Model file for the job. Use its own axes, mm. Coordinates: 2 decimals unless noted, no trailing zeros. Write each loop counter-clockwise with the first axis right and the second up, starting at its lowest first coordinate (ties: lowest second). Pieces come first, ordered by that corner, then holes.
Q1. Drill centre lines: probe 1 along X at (y, z) = (545, 8); probe 2 along Y at (x, z) = (-125, 9.25); probe 3 along Y at (x, z) = (-94, 8). Where is each one in solid material? Low to high.
Q2. Band-saw the part on D-D, the plane y = 595. Write the cut outline in (x, z), plus the area to 3 significant figures.
Q3. Band-saw the part on B-B, the plane z = 3. State how many separate pieces and enclosed holes the cut face has, plus the area to 3 significant figures.
Q4. Band-saw the part on C-C, the plane y = 490. Write the cut outline in (x, z), plus the area to 3 significant figures.
Q5. Pin check, flat tips, straight feed: P1, Ø1.2, axis at y = 595, z = 16, coming from the +X side; P2, Ø8, axis at x = -150.5, z = 5.5, coming from the -Y side (3 decimals); P3, Ø2.5, axis at x = -116.5, y = 593, coming from the +Z side. Stop position of each tip, or through.
Q6. Band-saw the part on A-A, the plane x = -125. Write the cut outline in (y, z), plus the area to 3 significant figures.
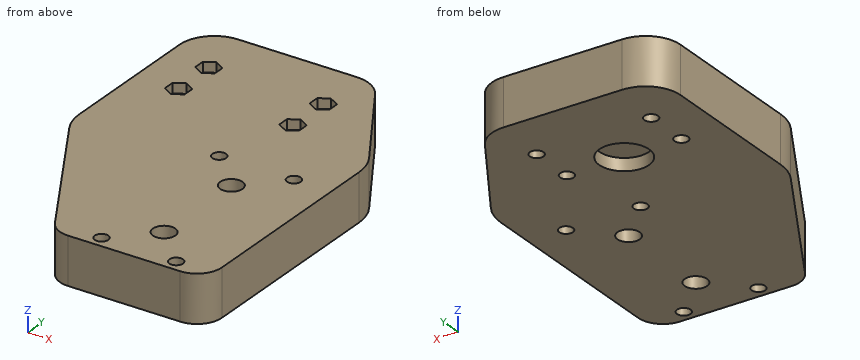
from build123d import *

# Parameters (mm, degrees)
BOSS_EXTRUDE1_DEPTH  = 19
FILLET1_R            = 10
M5_CLEARANCE_HOLE2_D = 5.5
M5_CLEARANCE_HOLE1_D = 5.5
FILLET2_R            = 4
BOSS_EXTRUDE2_DEPTH  = 19
M8_CLEARANCE_HOLE1_D = 9
CUT_EXTRUDE2_DEPTH   = 4
SKETCH16_R           = 10
CUT_EXTRUDE3_DEPTH   = 5


with BuildPart() as part:
    # Sketch1 → Boss-Extrude1 (new body)
    with BuildSketch(Plane.XY):
        with BuildLine():
            Line((-170.200000001, 540.824594888), (-129.309401077, 470))
            Line((-129.309401077, 470), (-93, 470))
            ThreePointArc((-93, 470), (-90.878679656, 470.878679656), (-90, 473))
            Line((-90, 473), (-90, 564.25527297))
            Line((-90, 564.25527297), (-116.225329238, 607))
            Line((-116.225329238, 607), (-170.200000001, 607))
            Line((-170.200000001, 607), (-170.200000001, 540.824594888))
        make_face()
    extrude(amount=BOSS_EXTRUDE1_DEPTH)

    # Fillet1
    fillet1_edges = [part.edges().sort_by_distance(p)[0] for p in [
        (-90, 564.25527297, 9.5),
        (-129.309401077, 470, 9.5),
        (-170.200000001, 540.824594888, 9.5),
    ]]
    fillet(fillet1_edges, radius=FILLET1_R)

    # M5 Clearance Hole2 (through all)
    with Locations(Plane(origin=(0, 0, 0), x_dir=(-1, 0, 0), z_dir=(0, 0, -1))):
        with Locations((117.000000001, 595), (117.000000001, 577), (163.000000001, 577), (163.000000001, 595)):
            Hole(M5_CLEARANCE_HOLE2_D / 2)

    # M5 Clearance Hole1 (through all)
    with Locations(Plane.XY.offset(19)):
        with Locations((-95, 545), (-125, 545), (-125, 475), (-95, 475), (-110, 490), (-110, 530)):
            Hole(M5_CLEARANCE_HOLE1_D / 2)

    # Fillet2
    fillet2_edges = [part.edges().sort_by_distance(p)[0] for p in [
        (-116.225329238, 607, 9.5),
        (-170.200000001, 607, 9.5),
    ]]
    fillet(fillet2_edges, radius=FILLET2_R)

    # Sketch11 → Boss-Extrude2 (add)
    with BuildSketch(Plane.XY.offset(19)):
        with BuildLine():
            ThreePointArc((-143.743157806, 475), (-140.082903769, 471.339745962), (-135.082903769, 470))
            Line((-135.082903769, 470), (-123.535898385, 470))
            ThreePointArc((-123.535898385, 470), (-128.535898385, 471.339745962), (-132.196152423, 475))
            Line((-132.196152423, 475), (-168.860254039, 538.504086813))
            ThreePointArc((-168.860254039, 538.504086813), (-169.859258264, 540.915896362), (-170.200000001, 543.504086813))
            Line((-170.200000001, 543.504086813), (-170.200000001, 603))
            ThreePointArc((-170.200000001, 603), (-169.028427125, 605.828427125), (-166.200000001, 607))
            Line((-166.200000001, 607), (-118.464037729, 607))
            ThreePointArc((-118.464037729, 607), (-116.510482263, 606.490504411), (-115.054590744, 605.091810521))
            Line((-115.054590744, 605.091810521), (-91.476382537, 566.661632408))
            ThreePointArc((-91.476382537, 566.661632408), (-90.37617086, 564.149073659), (-90, 561.432106106))
            Line((-90, 561.432106106), (-90, 473))
            ThreePointArc((-90, 473), (-90.878679656, 470.878679656), (-93, 470))
            Line((-93, 470), (-90, 470))
            ThreePointArc((-90, 470), (-82.928932188, 472.928932188), (-80, 480))
            Line((-80, 480), (-80, 561.432106106))
            ThreePointArc((-80, 561.432106106), (-80.75234172, 566.866041212), (-82.952765074, 571.89115871))
            Line((-82.952765074, 571.89115871), (-106.530973281, 610.321336823))
            ThreePointArc((-106.530973281, 610.321336823), (-111.626593598, 615.216765438), (-118.464037729, 617))
            Line((-118.464037729, 617), (-166.200000001, 617))
            ThreePointArc((-166.200000001, 617), (-176.099494937, 612.899494937), (-180.200000001, 603))
            Line((-180.200000001, 603), (-180.200000001, 543.504086813))
            ThreePointArc((-180.200000001, 543.504086813), (-179.518516526, 538.327705911), (-177.520508076, 533.504086813))
            Line((-177.520508076, 533.504086813), (-143.743157806, 475))
        make_face()
    extrude(amount=-BOSS_EXTRUDE2_DEPTH)

    # M8 Clearance Hole1 (through all)
    with Locations(Plane.XY.offset(19)):
        with Locations((-110, 530), (-110, 490)):
            Hole(M8_CLEARANCE_HOLE1_D / 2)

    # Sketch15 → Cut-Extrude2 (cut)
    with BuildSketch(Plane.XY.offset(19)):
        Polygon((-166.960000001, 579.286307066), (-166.960000001, 574.713692934), (-163.000000001, 572.427385868), (-159.040000001, 574.713692934), (-159.040000001, 579.286307066), (-163.000000001, 581.572614132), align=None)
        Polygon((-120.960000001, 579.286307066), (-120.960000001, 574.713692934), (-117.000000001, 572.427385868), (-113.040000001, 574.713692934), (-113.040000001, 579.286307066), (-117.000000001, 581.572614132), align=None)
        Polygon((-113.040000001, 592.713692934), (-117.000000001, 590.427385868), (-120.960000001, 592.713692934), (-120.960000001, 597.286307066), (-117.000000001, 599.572614132), (-113.040000001, 597.286307066), align=None)
        Polygon((-163.000000001, 590.427385868), (-166.960000001, 592.713692934), (-166.960000001, 597.286307066), (-163.000000001, 599.572614132), (-159.040000001, 597.286307066), (-159.040000001, 592.713692934), align=None)
    extrude(amount=-CUT_EXTRUDE2_DEPTH, mode=Mode.SUBTRACT)

    # Sketch16 → Cut-Extrude3 (cut)
    with BuildSketch(Plane(origin=(0, 0, 0), x_dir=(-1, 0, 0), z_dir=(0, 0, -1))):
        with Locations((140.000000001, 577)):
            Circle(SKETCH16_R)
    extrude(amount=-CUT_EXTRUDE3_DEPTH, mode=Mode.SUBTRACT)


solid = part.part
Answer sheet:
1. probe 1: x = -180.2 to -127.75, -122.25 to -97.75, -92.25 to -80
1. probe 2: y = 470 to 472.25, 477.75 to 542.25, 547.75 to 617
1. probe 3: y = 470 to 472.44, 477.56 to 542.44, 547.56 to 589.9
2. outline: (-180.2, 0) - (-165.75, 0) - (-165.75, 15) - (-166.96, 15) - (-166.96, 19) - (-180.2, 19) - close; (-160.25, 0) - (-119.75, 0) - (-119.75, 15) - (-120.96, 15) - (-120.96, 19) - (-159.04, 19) - (-159.04, 15) - (-160.25, 15) - close; (-114.25, 0) - (-97.13, 0) - (-97.13, 19) - (-113.04, 19) - (-113.04, 15) - (-114.25, 15) - close
2. area: 1,350 mm2
3. separate pieces: 1
3. enclosed holes: 11
3. area: 11,900 mm2
4. outline: (-152.4, 0) - (-114.5, 0) - (-114.5, 19) - (-152.4, 19) - close; (-105.5, 0) - (-80, 0) - (-80, 19) - (-105.5, 19) - close
4. area: 1,200 mm2
5. P1: stops at x = -96.76
5. P2: stops at y = 479.775
5. P3: stops at z = 15
6. outline: (470, 0) - (472.25, 0) - (472.25, 19) - (470, 19) - close; (477.75, 0) - (542.25, 0) - (542.25, 19) - (477.75, 19) - close; (547.75, 0) - (617, 0) - (617, 19) - (547.75, 19) - close
6. area: 2,580 mm2
